from build123d import *

# Parameters (mm, degrees)
SKETCH003_R       = 1.5
SKETCH003_R_2     = 1.6
PAD003_DEPTH      = 2
PAD003_DEPTH_BACK = 7
POCKET001_DEPTH   = 5
POCKET002_DEPTH   = 5


with BuildPart() as part:
    # Sketch003 → Pad003 (new body, two sides)
    with BuildSketch(Plane.XY) as pad003_sk:
        with BuildLine():
            ThreePointArc((-2.474873, 2.474874), (-2.474874, -2.474873), (2.474873, -2.474874))
            Line((2.474873, -2.474874), (8.520816, 3.571067))
            Line((20.621322, 3.571067), (8.520816, 3.571067))
            Line((26.667265, -2.474874), (20.621322, 3.571067))
            ThreePointArc((26.667265, -2.474874), (31.617012, -2.474873), (31.617011, 2.474874))
            Line((31.617011, 2.474874), (24.545942, 9.545941))
            ThreePointArc((24.545942, 9.545941), (23.410461, 10.304645), (22.071069, 10.571067))
            Line((22.071069, 10.571067), (7.071069, 10.571067))
            ThreePointArc((7.071069, 10.571067), (5.731677, 10.304645), (4.596196, 9.545941))
            Line((4.596196, 9.545941), (-2.474873, 2.474874))
        make_face()
        Circle(SKETCH003_R, mode=Mode.SUBTRACT)
        with Locations((29.142138, 0)):
            Circle(SKETCH003_R_2, mode=Mode.SUBTRACT)
    extrude(amount=-PAD003_DEPTH)
    extrude(pad003_sk.sketch, amount=PAD003_DEPTH_BACK)

    # Sketch006 → Pocket001 (cut)
    with BuildSketch(Plane.XY):
        with BuildLine():
            ThreePointArc((-2.651389, 2.284762), (-2.54902, -2.398437), (2.119285, -2.785432))
            Line((9.024723, 2.468542), (2.119285, -2.785432))
            Line((9.024723, 2.468542), (5.604523, 11.865468))
            Line((5.604523, 11.865468), (-2.651389, 2.284762))
        make_face()
    extrude(amount=POCKET001_DEPTH, mode=Mode.SUBTRACT)

    # Sketch008 → Pocket002 (cut)
    with BuildSketch(Plane(origin=(30, -0.7, 0), x_dir=(1, 0, 0), z_dir=(0, 0, 1))):
        with BuildLine():
            ThreePointArc((-2.085176, -2.811057), (2.596289, -2.347187), (2.587206, 2.357194))
            Line((-6.202528, 12.004617), (2.587206, 2.357194))
            Line((-9.195041, 2.462874), (-6.202528, 12.004617))
            Line((-9.195041, 2.462874), (-2.085176, -2.811057))
        make_face()
    extrude(amount=POCKET002_DEPTH, mode=Mode.SUBTRACT)


with BuildPart() as part_1:
    # Body001 placement: moved
    add(part.part.moved(Location((-30.2, 22, 0))))


solid = part_1.part
Input: part model. Units: mm. Frame: model coordinates. A direction names the side the tool comes from. Coordinates: 2 decimals unless noted, no trailing zeros. Loops run counter-clockwise (first coordinate to the right, second up) from the corner with the lowest first, then second, coordinate; pieces in that order, holes last. Notation, with made-up numbers: (57.5, 0) -> (78.5, 0) arc R25 ccw to (78.5, 19) -> close; hole circle Ø5 at (43.5, 40). An arc over 180 degrees is marked (long way). One line per item, written item: value.
(1) Draft query along X for faces 1 (the face through (-3, 25, 5)), 2 (the face through (-24.74, 22.51, 5.99)), 3 (the face through (-7.88, 28.59, 2.46)). Return one class per face: pulls with the +X half, pulls with the -X half, needs draft (parallel to the pull), parting line crosses it, or undercut.
Answer below:
face 1: needs draft
face 2: undercut
face 3: pulls with the +X half
(2) Cut plane C-C (x = -30.2). Output: boundary loops of the cut face in (y, z), then the cut area to 3 significant figures.
Answer below:
outline: (18.5, -2) -> (20.5, -2) -> (20.5, 0) -> (18.5, 0) -> close; (18.5, 5) -> (20.5, 5) -> (20.5, 7) -> (18.5, 7) -> close; (23.5, -2) -> (26.95, -2) -> (26.95, 0) -> (23.5, 0) -> close; (23.5, 5) -> (26.95, 5) -> (26.95, 7) -> (23.5, 7) -> close
area: 21.8 mm2
(3) Pin query (flat end, axial travel): pin 1 Ø5 at (x, y) = (-15.5, 23.5) entering from -Z; pin 2 Ø5 at (y, z) = (28, 3) entering from -X; pin 3 Ø2 at (y, z) = (23.5, -1) entering from -X; pin 4 Ø2.5 at (x, z) = (-15.5, 0.5) entering from -Y. Return the tip coordinate at first contact, or that it passes through.
Answer below:
pin 1: stops at z = -2
pin 2: stops at x = -30.65
pin 3: stops at x = -33.66
pin 4: stops at y = 25.57
(4) Ray query, line 1 along X through (y, z) = (22, 6.25); line 2 along Z through (x, y) = (-25.5, 23.5); line 3 along X through (y, z) = (21.75, 5.75). Return the intervals inside material, ascending.
Answer below:
line 1: x = -33.7 to -31.7, -28.7 to -25.25, -6.01 to -2.66, 0.54 to 2.44
line 2: z = -2 to 0, 5 to 7
line 3: x = -33.69 to -31.68, -28.72 to -25.5, -5.76 to -2.64, 0.52 to 2.43
(5) Cut plane D-D (z = 0.5). Output: boundary loops of the cut face in (x, y), then the cut area to 3 significant figures.
Answer below:
outline: (-24.08, 32.44) -> (-21.58, 25.57) -> (-9.58, 25.57) -> (-9.01, 25) -> (-6.72, 32.28) arc R3.5 ccw to (-8.13, 32.57) -> (-23.13, 32.57) arc R3.5 ccw to start
area: 106 mm2
(6) Set-up query: faces 4 (the face through (-28, 26, 5)), 5 (the face through (-16, 25.571, 2)), 6 (the face through (1.36, 19.47, -1.01)). Return all of +Z, -Z, +X, -X, +Y, -Y with unobstructed straight access to the full face (end or side cutting, diameter ignored); none if empty.
Answer below:
face 4: -X, -Y
face 5: +Z, -Z, -Y
face 6: +Z, -Z
(7) Cut plane B-B (y = 21.5). Give the number of separate pieces and of enclosed holes in the cut face, then the cut area to 3 significant figures.
Answer below:
separate pieces: 8
enclosed holes: 0
area: 39.8 mm2
